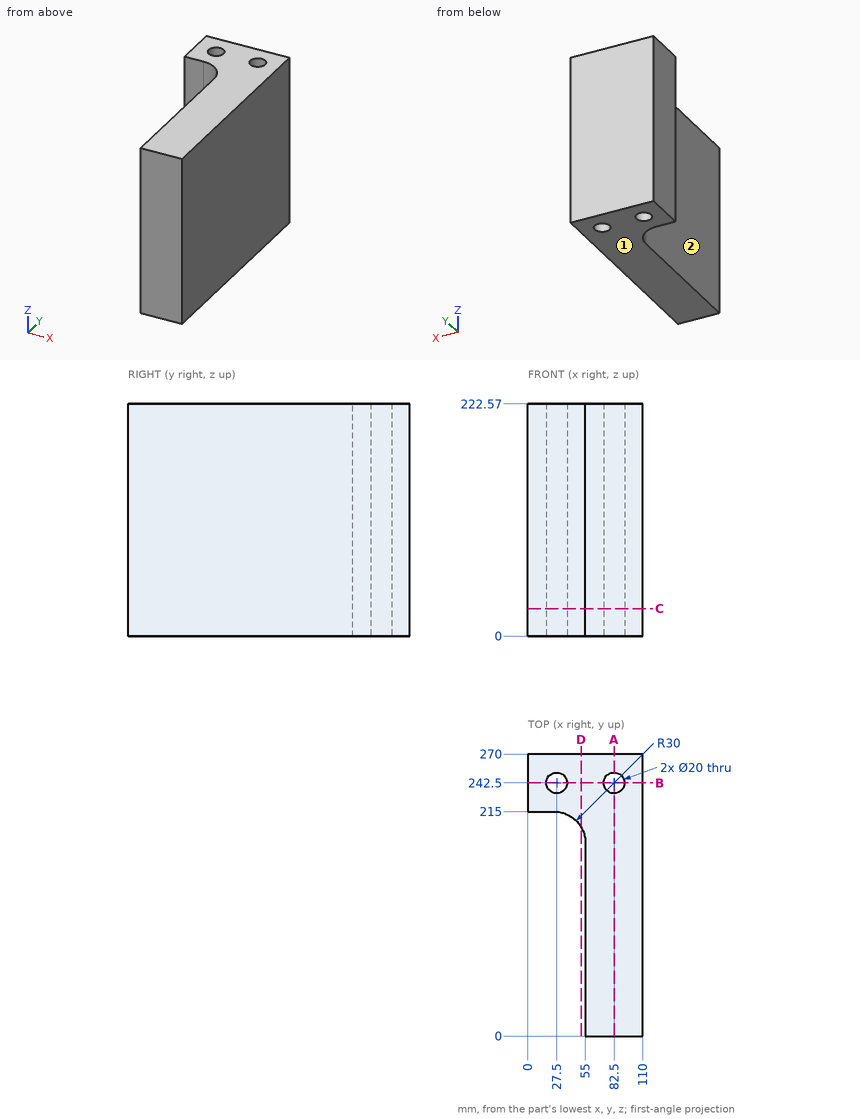
Geometry: see drawing. Coordinates: mm, zero at the bounding-box minimum. A direction names the side the tool comes from. Give positions to 0.01 mm unless a question says otherwise; leave off trailing zeros. Write each loop counter-clockwise with the first axis right and the second up, starting at its lowest first coordinate (ties: lowest second). Pieces come first, ordered by that corner, then holes. Notation, with made-up numbers: M 84.25,39 L 94.25,39 A21 cw 94.25,59 Z; hole C 17.25,-27 d3. An arc over 180 degrees is marked long. Return JSON: item names as keys, results as strings. Group by question number.
1) Cut plane C-C, the plane z = 26.5. Output: boundary loops of the cut face in (x, y).
2) Cut plane D-D, the plane x = 51. Output: boundary loops of the cut face in (y, z).
3) Cut plane A-A, the plane x = 82.5. Output: boundary loops of the cut face in (y, z).
4) Set-up query: the marked faces 1 and 2. Return all of +Z, -Z, +X, -X, +Y, -Y with unobstructed straight access to the full face (end or side cutting, diameter ignored); none if empty.
5) Ray query, L1, parallel to X at y = 242, z = 172; L2, parallel to Y at x = 82.5, z = 102.5; L3, parallel to Y at x = 27, z = 109. Return the intervals inside material, ascending.
6) First-contact query: pin 1 Ø1.5 at (y, z) = (35.5, 85) entering from -X; pin 2 Ø7.5 at (x, z) = (6.5, 72) entering from -Y; pin 3 Ø4 at (x, z) = (29.5, 123.5) entering from -Y. Flat tips, straight axial feed; report the tip coordinate or a pass-through.
7) Cut plane B-B, the plane y = 242.5. Output: boundary loops of the cut face in (x, z).
Data:
{
 "1": {"outline": "M 0,215 L 25,215 A30 cw 55,185 L 55,0 L 110,0 L 110,270 L 0,270 Z; hole C 27.5,242.5 d20; hole C 82.5,242.5 d20"},
 "2": {"outline": "M 199.97,0 L 270,0 L 270,222.57 L 199.97,222.57 Z"},
 "3": {"outline": "M 0,0 L 232.5,0 L 232.5,222.57 L 0,222.57 Z; M 252.5,0 L 270,0 L 270,222.57 L 252.5,222.57 Z"},
 "4": {"face 1": "-Z, +X, -X, +Y, -Y", "face 2": "+Z, -Z, -X, -Y"},
 "5": {"L1": "x = 0 to 17.51, 37.49 to 72.51, 92.49 to 110", "L2": "y = 0 to 232.5, 252.5 to 270", "L3": "y = 214.93 to 232.51, 252.49 to 270"},
 "6": {"pin 1": "stops at x = 55", "pin 2": "stops at y = 215", "pin 3": "stops at y = 214.29"},
 "7": {"outline": "M 0,0 L 17.5,0 L 17.5,222.57 L 0,222.57 Z; M 37.5,0 L 72.5,0 L 72.5,222.57 L 37.5,222.57 Z; M 92.5,0 L 110,0 L 110,222.57 L 92.5,222.57 Z"}
}
